Input: dimensioned drawing with shaded views. Units: mm. Origin: part minimum x, y, z. Round coordinates to 2 decimals unless told otherwise and drop trailing zeros. Loops run counter-clockwise (first coordinate to the right, second up) from the corner with the lowest first, then second, coordinate; pieces in that order, holes last. Notation, with made-up numbers: (-0.75, 4) - (26.25, 4) arc R27 ccw to (26.25, 25) - close; hole circle Ø11 at (23.25, 1.5). An arc over 180 degrees is marked (long way). Answer as CSV lines item,"result".
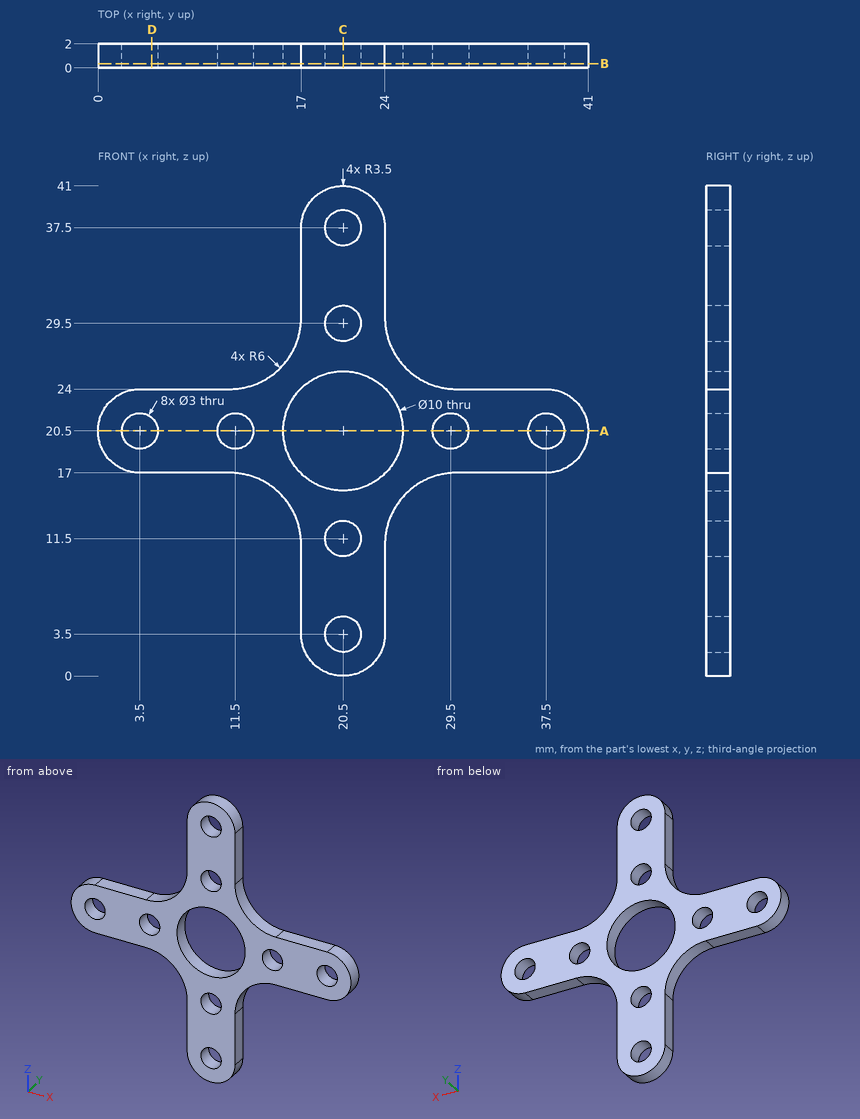
(1) Pin query (flat end, axial travel): P1, Ø1, axis at x = 7, y = 0.5, coming from the -Z side; P2, Ø0.6, axis at x = 34, y = 1, coming from the +Z side; P3, Ø1, axis at y = 1, z = 7.5, coming from the +X side. Return the tip coordinate at first contact, or that it passes through.
Findings below:
P1,"z = 17"
P2,"z = 24"
P3,"x = 24"
(2) Section A-A (z = 20.5). Output: boundary loops of the cut face in (x, y), and give its area (3 significant figures).
Findings below:
outline,"(0, 0) - (2, 0) - (2, 2) - (0, 2) - close; (5, 0) - (10, 0) - (10, 2) - (5, 2) - close; (13, 0) - (15.5, 0) - (15.5, 2) - (13, 2) - close; (25.5, 0) - (28, 0) - (28, 2) - (25.5, 2) - close; (31, 0) - (36, 0) - (36, 2) - (31, 2) - close; (39, 0) - (41, 0) - (41, 2) - (39, 2) - close"
area,"38.0 mm2"
(3) Material intervals for line 1 along Z through (x, y) = (20.5, 0.6); line 2 along Z through (x, y) = (21, 1.25), sorted ascending.
Findings below:
line 1,"0 to 2, 5 to 10, 13 to 15.5, 25.5 to 28, 31 to 36, 39 to 41"
line 2,"0.04 to 2.09, 4.91 to 10.09, 12.91 to 15.53, 25.47 to 28.09, 30.91 to 36.09, 38.91 to 40.96"
(4) Section C-C (x = 20.5). Output: boundary loops of the cut face in (y, z), and give its area (3 significant figures).
Findings below:
outline,"(0, 0) - (2, 0) - (2, 2) - (0, 2) - close; (0, 5) - (2, 5) - (2, 10) - (0, 10) - close; (0, 13) - (2, 13) - (2, 15.5) - (0, 15.5) - close; (0, 25.5) - (2, 25.5) - (2, 28) - (0, 28) - close; (0, 31) - (2, 31) - (2, 36) - (0, 36) - close; (0, 39) - (2, 39) - (2, 41) - (0, 41) - close"
area,"38.0 mm2"
(5) Section B-B (y = 0.35). Give the number of separate pieces and of enclosed holes in the cut face, and give its area (3 significant figures).
Findings below:
separate pieces,"1"
enclosed holes,"9"
area,"400 mm2"
(6) Section D-D (x = 4.5). Output: boundary loops of the cut face in (y, z), and give its area (3 significant figures).
Findings below:
outline,"(0, 17) - (2, 17) - (2, 19.38) - (0, 19.38) - close; (0, 21.62) - (2, 21.62) - (2, 24) - (0, 24) - close"
area,"9.53 mm2"
